from build123d import *

# Parameters (mm, degrees)
SKETCH_W                      = 19.6
SKETCH_H                      = 17
PAD_DEPTH                     = 15.7
SKETCH001_W                   = 19.6
SKETCH001_H                   = 8.5
POCKET_DEPTH                  = 0.25
SKETCH002_W                   = 16.5
SKETCH002_H                   = 8.5
POCKET001_DEPTH               = 0.5
SKETCH008_W                   = 19.6
SKETCH008_H                   = 17
POCKET002_DEPTH               = 0.5
SKETCH009_W                   = 17
SKETCH009_H                   = 1.5
POCKET003_DEPTH               = 0.5
SKETCH010_W                   = 2
SKETCH010_H                   = 5.2
POCKET004_DEPTH               = 0.5
SKETCH010_MIRRORED005_2_W     = 2
SKETCH010_MIRRORED005_2_H     = 5.2
POCKET004_MIRRORED005_2_DEPTH = 0.5
SKETCH024_W                   = 19.6
SKETCH024_H                   = 17
POCKET006_DEPTH               = 1.2
SKETCH025_W                   = 16
SKETCH025_H                   = 1
PAD011_DEPTH                  = 1.2
SKETCH038_W                   = 1
SKETCH038_H                   = 1
PAD014_DEPTH                  = 1.2
SKETCH038_MIRRORED012_2_W     = 1
SKETCH038_MIRRORED012_2_H     = 1
PAD014_MIRRORED012_2_DEPTH    = 1.2
FILLET003_R                   = 0.5
FILLET004_R                   = 0.25


with BuildPart() as part:
    # Sketch → Pad (new body)
    with BuildSketch(Plane.XY):
        Rectangle(SKETCH_W, SKETCH_H)
    extrude(amount=PAD_DEPTH)

    # Sketch001 (on Face3 of Pad) → Pocket (cut)
    with BuildSketch(Plane.XZ.offset(8.5)):
        with Locations((0, 4.25)):
            Rectangle(SKETCH001_W, SKETCH001_H)
    pocket = extrude(amount=-POCKET_DEPTH, mode=Mode.SUBTRACT)

    # Mirrored: Pocket across XZ
    add(pocket.mirror(Plane.XZ), mode=Mode.SUBTRACT)

    # Sketch002 (on Face5 of Mirrored) → Pocket001 (cut)
    with BuildSketch(Plane(origin=(-9.8, 0, 0), x_dir=(0, -1, 0), z_dir=(-1, 0, 0))):
        with Locations((0, 4.25)):
            Rectangle(SKETCH002_W, SKETCH002_H)
    pocket001 = extrude(amount=-POCKET001_DEPTH, mode=Mode.SUBTRACT)

    # Mirrored001: Pocket001 across YZ
    add(pocket001.mirror(Plane.YZ), mode=Mode.SUBTRACT)

    # Sketch008 (on Face4 of Mirrored001) → Pocket002 (cut)
    with BuildSketch(Plane.XY.offset(15.7)):
        Rectangle(SKETCH008_W, SKETCH008_H)
    extrude(amount=-POCKET002_DEPTH, mode=Mode.SUBTRACT)

    # Sketch009 (on Face4 of Pocket002) → Pocket003 (cut)
    with BuildSketch(Plane(origin=(-9.8, 0, 0), x_dir=(0, -1, 0), z_dir=(-1, 0, 0))):
        with Locations((0, 14.45)):
            Rectangle(SKETCH009_W, SKETCH009_H)
    pocket003 = extrude(amount=-POCKET003_DEPTH, mode=Mode.SUBTRACT)

    # Mirrored004: Pocket003 across YZ
    add(pocket003.mirror(Plane.YZ), mode=Mode.SUBTRACT)

    # Sketch010 (on Face8 of Mirrored004) → Pocket004 (cut)
    with BuildSketch(Plane(origin=(-9.8, 0, 0), x_dir=(0, -1, 0), z_dir=(-1, 0, 0))):
        with Locations((-5.5, 11.1)):
            Rectangle(SKETCH010_W, SKETCH010_H)
    pocket004 = extrude(amount=-POCKET004_DEPTH, mode=Mode.SUBTRACT)

    # Sketch010 Mirrored005 2 → Pocket004 Mirrored005 2 (cut)
    with BuildSketch(Plane.YZ.offset(-9.8)):
        with Locations((-5.5, 11.1)):
            Rectangle(SKETCH010_MIRRORED005_2_W, SKETCH010_MIRRORED005_2_H)
    pocket004_mirrored005_2 = extrude(amount=POCKET004_MIRRORED005_2_DEPTH, mode=Mode.SUBTRACT)

    # Mirrored006: Pocket004, Pocket004 Mirrored005 2 across YZ
    add(pocket004.mirror(Plane.YZ), mode=Mode.SUBTRACT)
    add(pocket004_mirrored005_2.mirror(Plane.YZ), mode=Mode.SUBTRACT)

    # Sketch024 (on Face13 of MultiTransform) → Pocket006 (cut)
    with BuildSketch(Plane(origin=(0, 0, 0), x_dir=(1, 0, 0), z_dir=(0, 0, -1))):
        Rectangle(SKETCH024_W, SKETCH024_H)
    extrude(amount=-POCKET006_DEPTH, mode=Mode.SUBTRACT)

    # Sketch025 (on Face12 of Pocket006) → Pad011 (join)
    with BuildSketch(Plane(origin=(0, 0, 1.2), x_dir=(1, 0, 0), z_dir=(0, 0, -1))):
        with Locations((0, 2.4)):
            Rectangle(SKETCH025_W, SKETCH025_H)
        with Locations((0, -2.4)):
            Rectangle(SKETCH025_W, SKETCH025_H)
    extrude(amount=PAD011_DEPTH)

    # Sketch038 (on Face12 of Pad011) → Pad014 (join)
    with BuildSketch(Plane(origin=(0, 0, 1.2), x_dir=(1, 0, 0), z_dir=(0, 0, -1))):
        with Locations((-8.8, 7.75)):
            Rectangle(SKETCH038_W, SKETCH038_H)
    pad014 = extrude(amount=PAD014_DEPTH)

    # Sketch038 Mirrored012 2 → Pad014 Mirrored012 2 (add)
    with BuildSketch(Plane.XY.offset(1.2)):
        with Locations((-8.8, 7.75)):
            Rectangle(SKETCH038_MIRRORED012_2_W, SKETCH038_MIRRORED012_2_H)
    pad014_mirrored012_2 = extrude(amount=-PAD014_MIRRORED012_2_DEPTH)

    # Mirrored013: Pad014, Pad014 Mirrored012 2 across YZ
    add(pad014.mirror(Plane.YZ))
    add(pad014_mirrored012_2.mirror(Plane.YZ))

    # Fillet003
    fillet003_edges = [part.edges().sort_by_distance(p)[0] for p in [
        (9.3, -8.25, 4.25),
        (-9.3, -8.25, 4.25),
        (9.3, 8.25, 4.25),
        (-9.3, 8.25, 4.25),
    ]]
    fillet(fillet003_edges, radius=FILLET003_R)

    # Fillet004
    fillet004_edges = [part.edges().sort_by_distance(p)[0] for p in [
        (-9.8, 8.5, 11.1),
        (-9.8, -8.5, 11.1),
        (9.8, 8.5, 11.1),
        (9.8, -8.5, 11.1),
    ]]
    fillet(fillet004_edges, radius=FILLET004_R)


solid = part.part
Verification items for the finished model (mm, model axes). A direction names the side the tool comes from. Give positions to 0.01 mm unless a question says otherwise; leave off trailing zeros. Loops run counter-clockwise (first coordinate to the right, second up) from the corner with the lowest first, then second, coordinate; pieces in that order, holes last.
1) Sectioned sample at B-B, the plane x = 4.5. Enter the section's corners in (y, z).
2) Set-up check for faces 5 (the flat face through (8.3, 8, 1)), 6 (the flat face through (9.8, -7, 11)), 7 (the flat face through (9, -7.25, 1)), 8 (the flat face through (-9, -8, 0)), 9 (the flat face through (0, -2.9, 1)): record each of +Z, -Z, +X, -X, +Y, -Y from which the full face is reachable in a straight line by a thin tool's end or side.
3) Thickness scan on line 1 along X through (y, z) = (-5.25, 12.75); line 2 along Y through (x, z) = (-0.75, 8); line 3 along Z through (x, y) = (-0.5, 0.75). Record the ranges inside material, lowest first.
4) Depth check by flat-ended pin: pin 1 Ø1 at (y, z) = (-3, 5.5) entering from +X; pin 2 Ø4.5 at (y, z) = (-3, 7.5) entering from +X; pin 3 Ø0.5 at (x, z) = (9, 0.5) entering from -Y; pin 4 Ø1.3 at (x, z) = (0, 0.5) entering from -Y. Enter the tip coordinate at first touch or a pass-through.
5) Sectioned sample at C-C, the plane z = 7.25. Enter the section's corners in (x, y).
6) Draft check along X on faces 1 (the flat face through (-9.8, 0, 11)), 2 (the flat face through (-8.3, 8, 1)), 3 (the flat face through (-8.3, -8, 1)), 4 (the flat face through (-0.1, 2.4, 0)). Enter one of: pulls with the +X half, pulls with the -X half, needs draft (parallel to the pull), parting line crosses it, or undercut.
7) Sectioned sample at A-A, the plane y = -2.25. Enter the section's corners in (x, z).
8) Sectioned sample at D-D, the plane y = 6.75. Enter the section's corners in (x, z).
Answers:
1. outline: (-8.5, 8.5) - (-8.25, 8.5) - (-8.25, 1.2) - (-2.9, 1.2) - (-2.9, 0) - (-1.9, 0) - (-1.9, 1.2) - (1.9, 1.2) - (1.9, 0) - (2.9, 0) - (2.9, 1.2) - (8.25, 1.2) - (8.25, 8.5) - (8.5, 8.5) - (8.5, 15.2) - (-8.5, 15.2) - close
2. face 5: -Z, +Y, -Y
2. face 6: +Z, -Z, +X, +Y, -Y
2. face 7: -Z, +X, -X
2. face 8: -Z, +X, -X, +Y, -Y
2. face 9: -Z, +X, -X, -Y
3. line 1: x = -9.3 to 9.3
3. line 2: y = -8.25 to 8.25
3. line 3: z = 1.2 to 15.2
4. pin 1: stops at x = 9.3
4. pin 2: stops at x = 9.8
4. pin 3: stops at y = -8.25
4. pin 4: stops at y = -2.9
5. outline: (-9.3, -7.75) arc R0.5 ccw to (-8.8, -8.25) - (8.8, -8.25) arc R0.5 ccw to (9.3, -7.75) - (9.3, 7.75) arc R0.5 ccw to (8.8, 8.25) - (-8.8, 8.25) arc R0.5 ccw to (-9.3, 7.75) - close
6. face 1: pulls with the -X half
6. face 2: undercut
6. face 3: undercut
6. face 4: needs draft
7. outline: (-9.8, 8.5) - (-9.3, 8.5) - (-9.3, 1.2) - (-8, 1.2) - (-8, 0) - (8, 0) - (8, 1.2) - (9.3, 1.2) - (9.3, 8.5) - (9.8, 8.5) - (9.8, 13.7) - (9.3, 13.7) - (9.3, 15.2) - (-9.3, 15.2) - (-9.3, 13.7) - (-9.8, 13.7) - close
8. outline: (-9.8, 8.5) - (-9.3, 8.5) - (-9.3, 1.2) - (9.3, 1.2) - (9.3, 8.5) - (9.8, 8.5) - (9.8, 13.7) - (9.3, 13.7) - (9.3, 15.2) - (-9.3, 15.2) - (-9.3, 13.7) - (-9.8, 13.7) - close
